Geometry: final body of the model. Coordinates: model frame, mm. Coordinates: 2 decimals unless noted, no trailing zeros. Write each loop counter-clockwise with the first axis right and the second up, starting at its lowest first coordinate (ties: lowest second). Pieces come first, ordered by that corner, then holes. Notation, with made-up numbers: (29.5, -18) -> (33.5, -18) arc R23 ccw to (33.5, -10) -> close; hole circle Ø3 at (-16, 62.5). An arc over 180 degrees is marked (long way). One line per item, written item: value.
```python
from build123d import *

# Parameters (mm, degrees)
BOSS_EXTRU_1_DEPTH      = 10
ESQUISSE3_R             = 5
ENL_V_MAT_EXTRU_1_DEPTH = 10
CHANFREIN1_SIZE         = 3
ESQUISSE4_R             = 20
ENL_V_MAT_EXTRU_2_DEPTH = 10
CHANFREIN2_SIZE         = 3


with BuildPart() as part:
    # Esquisse1 → Boss.-Extru.1 (new body)
    with BuildSketch(Plane.XY):
        with BuildLine():
            Line((-224.722989012, -199.030461543), (225.277010988, -199.030461543))
            ThreePointArc((225.277010988, -199.030461543), (242.954680517, -191.708131073), (250.277010988, -174.030461543))
            Line((250.277010988, -174.030461543), (250.277010988, 175.969538457))
            ThreePointArc((250.277010988, 175.969538457), (242.954680517, 193.647207986), (225.277010988, 200.969538457))
            Line((225.277010988, 200.969538457), (-224.722989012, 200.969538457))
            ThreePointArc((-224.722989012, 200.969538457), (-242.400658542, 193.647207986), (-249.722989012, 175.969538457))
            Line((-249.722989012, 175.969538457), (-249.722989012, -174.030461543))
            ThreePointArc((-249.722989012, -174.030461543), (-242.400658542, -191.708131073), (-224.722989012, -199.030461543))
        make_face()
    extrude(amount=BOSS_EXTRU_1_DEPTH)

    # Esquisse3 → Enlèv. mat.-Extru.1 (cut)
    with BuildSketch(Plane.XY.offset(10)):
        with Locations((-224.722989012, -174.030461543)):
            Circle(ESQUISSE3_R)
        with Locations((225.277010988, -174.030461543)):
            Circle(ESQUISSE3_R)
        with Locations((225.277010988, 175.969538457)):
            Circle(ESQUISSE3_R)
        with Locations((-224.722989012, 175.969538457)):
            Circle(ESQUISSE3_R)
    extrude(amount=-ENL_V_MAT_EXTRU_1_DEPTH, mode=Mode.SUBTRACT)

    # Chanfrein1
    chanfrein1_edges = [part.edges().sort_by_distance(p)[0] for p in [
        (-229.722989012, 175.969538457, 10),
        (220.277010988, 175.969538457, 10),
        (220.277010988, -174.030461543, 10),
        (-229.722989012, -174.030461543, 10),
    ]]
    chamfer(chanfrein1_edges, length=CHANFREIN1_SIZE)

    # Esquisse4 → Enlèv. mat.-Extru.2 (cut)
    with BuildSketch(Plane.XY.offset(10)):
        with Locations((0, -121.160461543)):
            Circle(ESQUISSE4_R)
    extrude(amount=-ENL_V_MAT_EXTRU_2_DEPTH, mode=Mode.SUBTRACT)

    # Chanfrein2
    chanfrein2_edges = [part.edges().sort_by_distance(p)[0] for p in [
        (-20, -121.160461543, 0),
        (-20, -121.160461543, 10),
    ]]
    chamfer(chanfrein2_edges, length=CHANFREIN2_SIZE)


solid = part.part
```
(1) Line query: line 1 (X direction, y = 179, z = 9.5); line 2 (X direction, y = 178, z = 0.5); line 3 (Y direction, x = -8, z = 7.25). Output: solid intervals per line, ascending. Write a range as [from, to].
Responses:
line 1: x = [-249.54, -231.58], [-217.86, 218.42], [232.14, 250.09]
line 2: x = [-249.64, -229.29], [-220.15, 220.71], [229.85, 250.19]
line 3: y = [-199.03, -139.76], [-102.56, 200.97]
(2) Pull-direction query (X, two-part tool) for faces 1 (the flat face through (-3, 4, 0)), 2 (the conical face through (-228.81, 172.84, 7.15)), 3 (the cylindrical face through (-242.205, 193.841, 4.93)); classes: released by +X, released by -X, zero draft, split by the parting line, or undercut.
Responses:
face 1: zero draft
face 2: undercut
face 3: released by -X
(3) First-contact query: pin 1 (6 mm diameter, centred on x = -224.72, y = 175.97, fed in from -Z); pin 2 (13 mm diameter, centred on x = -224.72, y = -174.03, fed in from +Z). Flat tips, straight axial feed; report the tip coordinate or a pass-through.
Responses:
pin 1: passes through
pin 2: stops at z = 8.5
(4) Section A-A (x = 0). Return the cut outline in (y, z), then the cut area to 3 significant figures.
Responses:
outline: (-199.03, 0) -> (-144.16, 0) -> (-141.16, 3) -> (-141.16, 7) -> (-144.16, 10) -> (-199.03, 10) -> close; (-101.16, 3) -> (-98.16, 0) -> (200.97, 0) -> (200.97, 10) -> (-98.16, 10) -> (-101.16, 7) -> close
area: 3,580 mm2
